Could you check a few things on this model? Use its own coordinates, in mm. A direction names the side the tool comes from. Give positions to 0.01 mm unless a question says otherwise; leave off trailing zeros. Loops run counter-clockwise (first coordinate to the right, second up) from the corner with the lowest first, then second, coordinate; pieces in that order, holes last.
1. For faces 1 (the cylindrical face through (21.18, -0.45, 39.45)), 2 (the flat face through (16, -11.5, 18)), 3 (the flat face through (6.5, -7, 21)), 4 (the cylindrical face through (25.07, -16.05, 22.03)), which set-ups out of +Z, -Z, +X, -X, +Y, -Y let a thin tool reach every point of the face, with its end or its side?
2. Imagine slicing it at D-D (x = 16). List the corners of the cut face in (y, z) for me, plus the area to 3 significant figures.
3. For P1, Ø6, axis at x = 17.5, y = -7, coming from the -Z side; P2, Ø12, axis at x = 16.5, z = 20, coming from the +Y side; P3, Ø0.9, axis at y = -3.5, z = 40, coming from the +X side, each with a flat end and sliding along its axis, tell me the tip position at first contact or that it passes through.
4. I need wall thicknesses on line 1 along Y through (x, z) = (3.75, 1.4); line 2 along X through (y, z) = (-2.5, 19); line 3 along Y through (x, z) = (14, 28). Which ranges of each line are inside material? Lowest first, please.
5. Imagine slicing it at B-B (y = -3.5). List the corners of the cut face in (x, z) for me, plus the area to 3 significant figures.
6. Thinking about a two-plate mould opening in X: for faces 5 (the cylindrical face through (16.1, -9.25, 39.55)), 6 (the cylindrical face through (25.07, -7.4, 42.55)), 7 (the cylindrical face through (6.93, -7.6, 42.55)), 8 (the flat face through (16, -12, 0)), which applies, +X half, -X half, draft (parallel to the pull), parting line (faces both ways), or undercut?
7. Imagine slicing it at A-A (x = 28.25). List the corners of the cut face in (y, z) for me.
8. Imagine slicing it at C-C (z = 23). List the corners of the cut face in (x, y) for me, plus the area to 3 significant figures.
```python
from build123d import *

# Parameters (mm, degrees)
F0_R     = 1.75
F1_DEPTH = 2
F3_DEPTH = 41
F5_DEPTH = 7
F6_R     = 1.5


with BuildPart() as f1:
    # F0 (on Top) → F1 (new body)
    with BuildSketch(Plane.XY):
        Polygon((0, 0), (0, -16.5), (32, -16.5), (32, 0), (24.5, 0), (24.5, -11.5), (7.5, -11.5), (7.5, 0), align=None)
        with Locations((3.75, -4.75)):
            Circle(F0_R, mode=Mode.SUBTRACT)
        with Locations((28.25, -4.75)):
            Circle(F0_R, mode=Mode.SUBTRACT)
    extrude(amount=F1_DEPTH)

    # F2 (on face) → F3 (join)
    with BuildSketch(Plane.XY.offset(2)):
        Polygon((7.5, -11.5), (7.5, 0), (6.5, 0), (6.5, -16.5), (25.5, -16.5), (25.5, 0), (24.5, 0), (24.5, -11.5), align=None)
    extrude(amount=F3_DEPTH)

    # F4 (on face) → F5 (join)
    with BuildSketch(Plane.XY.offset(43)):
        with BuildLine():
            Line((20.75, 0), (20.75, -4.5))
            ThreePointArc((20.75, -4.5), (16, -9.25), (11.25, -4.5))
            Line((11.25, -4.5), (11.25, 0))
            Line((11.25, 0), (7.5, 0))
            Line((7.5, 0), (7.5, -11.5))
            Line((7.5, -11.5), (24.5, -11.5))
            Line((24.5, -11.5), (24.5, 0))
            Line((24.5, 0), (20.75, 0))
        make_face()
    extrude(amount=-F5_DEPTH)

    # F6
    f6_edges = [f1.edges().sort_by_distance(p)[0] for p in [
        (25.5, -8.25, 43),
        (11.25, 0, 39.5),
        (20.75, 0, 39.5),
        (6.5, -8.25, 43),
        (6.5, -16.5, 22.5),
        (16, -16.5, 43),
        (25.5, -16.5, 22.5),
        (32, -16.5, 1),
        (32, 0, 1),
        (0, -16.5, 1),
        (0, 0, 1),
    ]]
    fillet(f6_edges, radius=F6_R)


solid = f1.part
```
Derived:
1. face 1: +Z, -Z, +Y
1. face 2: -Z, +Y
1. face 3: +Z, -X, +Y, -Y
1. face 4: +Z, +X, -Y
2. outline: (-16.5, 0) - (-11.5, 0) - (-11.5, 36) - (-9.25, 36) - (-9.25, 43) - (-15, 43) arc R1.5 ccw to (-16.5, 41.5) - close
2. area: 230 mm2
3. P1: stops at z = 36
3. P2: stops at y = -11.5
3. P3: stops at x = 25.5
4. line 1: y = -16.5 to -6.5, -3 to 0
4. line 2: x = 6.5 to 7.5, 24.5 to 25.5
4. line 3: y = -16.5 to -11.5
5. outline: (0, 0) - (2.53, 0) - (2.53, 2) - (0, 2) - close; (4.97, 0) - (7.5, 0) - (7.5, 36) - (11.25, 36) - (11.25, 43) - (8, 43) arc R1.5 ccw to (6.5, 41.5) - (6.5, 2) - (4.97, 2) - close; (20.75, 36) - (24.5, 36) - (24.5, 0) - (27.03, 0) - (27.03, 2) - (25.5, 2) - (25.5, 41.5) arc R1.5 ccw to (24, 43) - (20.75, 43) - close; (29.47, 0) - (32, 0) - (32, 2) - (29.47, 2) - close
5. area: 154 mm2
6. face 5: undercut
6. face 6: +X half
6. face 7: -X half
6. face 8: draft
7. outline: (-16.5, 0) - (-6.5, 0) - (-6.5, 2) - (-16.5, 2) - close; (-3, 0) - (0, 0) - (0, 2) - (-3, 2) - close
8. outline: (6.5, -15) arc R1.5 ccw to (8, -16.5) - (24, -16.5) arc R1.5 ccw to (25.5, -15) - (25.5, 0) - (24.5, 0) - (24.5, -11.5) - (7.5, -11.5) - (7.5, 0) - (6.5, 0) - close
8. area: 117 mm2
